```python
from build123d import *

# Parameters (mm, degrees)
SKETCH2_W           = 2.54
SKETCH2_H           = 14.2875
CUT_EXTRUDE1_DEPTH  = 16.757342995
SKETCH3_W           = 1.5875
SKETCH3_H           = 7.9375
SKETCH3_W_2         = 4.7625
SKETCH3_H_2         = 4.7625
BOSS_EXTRUDE2_DEPTH = 3.175
SKETCH4_R           = 1.5875
CUT_EXTRUDE2_DEPTH  = 18.768884025
CHAMFER2_SIZE       = 0.79375
FILLET3_R           = 3.175


with BuildPart() as part:
    # Sketch1 → Revolve1 (revolve)
    with BuildSketch(Plane.XY, mode=Mode.PRIVATE) as revolve1_sk:
        Polygon((1.5875, 7.9375), (1.5875, 0), (3.0988, 0), (3.0988, 6.35), (4.699, 6.35), (4.699, 14.2875), (3.1115, 14.2875), (3.1115, 7.9375), align=None)
    revolve(revolve1_sk.sketch.rotate(Axis((0, 0.120875177, 0), (0, -1, 0)), 180), axis=Axis((0, 0.120875177, 0), (0, -1, 0)))

    # Sketch2 → Cut-Extrude1 (cut, through all)
    with BuildSketch(Plane.XY):
        with Locations((0, 7.14375)):
            Rectangle(SKETCH2_W, SKETCH2_H)
    extrude(amount=CUT_EXTRUDE1_DEPTH, mode=Mode.SUBTRACT)

    # Sketch3 → Boss-Extrude2 (add, symmetric)
    # profile 1 of 3: a face of its own
    with BuildSketch(Plane(origin=(0, 0, 0), x_dir=(0, 0, -1), z_dir=(1, 0, 0))):
        with Locations((3.90525, 10.31875)):
            Rectangle(SKETCH3_W, SKETCH3_H)
    # profile 2 of 3: a face of its own
    with BuildSketch(Plane(origin=(0, 0, 0), x_dir=(0, 0, -1), z_dir=(1, 0, 0))):
        with Locations((7.08025, 10.31875)):
            Rectangle(SKETCH3_W_2, SKETCH3_H)
        with Locations((7.08025, 10.31875)):
            Rectangle(SKETCH3_W, SKETCH3_H_2, mode=Mode.SUBTRACT)
    # profile 3 of 3: a face of its own
    with BuildSketch(Plane(origin=(0, 0, 0), x_dir=(0, 0, -1), z_dir=(1, 0, 0))):
        with Locations((7.08025, 10.31875)):
            Rectangle(SKETCH3_W, SKETCH3_H_2)
    extrude(amount=BOSS_EXTRUDE2_DEPTH, both=True)

    # Sketch4 → Cut-Extrude2 (cut, through all)
    with BuildSketch(Plane(origin=(0, 14.2875, 0), x_dir=(1, 0, 0), z_dir=(0, 1, 0))):
        with Locations(Location((0, 6.2865, 0), (0, 0, 180))):
            Circle(SKETCH4_R)
    extrude(amount=-CUT_EXTRUDE2_DEPTH, mode=Mode.SUBTRACT)

    # Chamfer2
    chamfer2_edges = [part.edges().sort_by_distance(p)[0] for p in [
        (0, 14.2875, -3.1115),
        (0, 0, -3.0988),
        (1.5875, 6.35, -6.2865),
        (1.5875, 14.2875, -6.2865),
    ]]
    chamfer(chamfer2_edges, length=CHAMFER2_SIZE - 0.0001)  # a hair under: the kernel refuses the full size

    # Fillet3
    fillet3_edges = [part.edges().sort_by_distance(p)[0] for p in [
        (3.175, 10.31875, -3.464098151),
        (-3.175, 10.31875, -3.464098151),
        (-3.175, 10.31875, -9.4615),
        (3.175, 10.31875, -9.4615),
    ]]
    fillet(fillet3_edges, radius=FILLET3_R - 0.0001)  # a hair under: the kernel refuses the full size


solid = part.part
```
Check sheet for the modelled part. Datum: model origin and axes. Units: mm. A direction names the side the tool comes from. Coordinates: 2 decimals unless noted, no trailing zeros. Loops run counter-clockwise (first coordinate to the right, second up) from the corner with the lowest first, then second, coordinate; pieces in that order, holes last.
1) Gauge pin test, flat ends, axial feed: pin 1 (4 mm diameter, centred on y = 9.5, z = 2.5, fed in from +X); pin 2 (2 mm diameter, centred on x = -3.5, z = -3.5, fed in from -Y); pin 3 (3 mm diameter, centred on x = 1, y = 9.5, fed in from +Z); pin 4 (3 mm diameter, centred on x = 0, z = 0, fed in from -Y). Record the tip position at first contact, or that the pin passes through.
2) Sectioned sample at C-C (y = 2.25). Record the boundary of the cut face in (x, z) (1 decimal), and give its area (3 significant figures).
3) Release check for a two-part mould opening along Z. For faces 1 (the face through (-3.33, 10.37, -3.68)), 2 (the face through (0.344, 10.363, -7.836)), 3 (the face through (-3.175, 10, -5)) record: released by +Z, released by -Z, zero draft, split by the parting line, or undercut.
4) Sectioned sample at A-A (z = 0). Record the boundary of the cut face in (x, y).
5) Access from +Z, -Z, +X, -X, +Y, -Y to the whole of each face (thin tool, end or side, straight path). Record for faces 4 (the face through (3.33, 10.37, -3.68)), 5 (the face through (-0.118, 3.611, -3.097)), 6 (the face through (-0.12, 10.68, -3.11)), 7 (the face through (-1.27, 7, 3)), 8 (the face through (-4.42, 10.37, 1.59)).
6) Material ranges on probe 1 along Z at (x, y) = (0, 11.25); probe 2 along X at (y, z) = (9.5, 0); probe 3 along X at (y, z) = (3.75, 0), recorded low to high.
Check sheet entries:
1. pin 1: stops at x = 4.67
1. pin 2: stops at y = 6.35
1. pin 3: stops at z = 4.52
1. pin 4: passes through
2. outline: (-1.3, 1) - (-1.3, 2.8) arc R3.1 ccw (long way) to (1.3, 2.8) - (1.3, 1) arc R1.6 cw (long way) to start
2. area: 18.2 mm2
3. face 1: released by -Z
3. face 2: undercut
3. face 3: zero draft
4. outline: (-4.7, 6.35) - (-3.1, 6.35) - (-3.1, 0.79) - (-2.31, 0) - (-1.59, 0) - (-1.59, 7.94) - (-3.11, 7.94) - (-3.11, 13.49) - (-3.91, 14.29) - (-4.7, 14.29) - close; (1.59, 0) - (2.31, 0) - (3.1, 0.79) - (3.1, 6.35) - (4.7, 6.35) - (4.7, 14.29) - (3.91, 14.29) - (3.11, 13.49) - (3.11, 7.94) - (1.59, 7.94) - close
5. face 4: -Z, +X, +Y, -Y
5. face 5: -Y
5. face 6: +Y
5. face 7: +Z, +Y, -Y
5. face 8: -X, +Y, -Y
6. probe 1: z = -9.46 to -7.87, -4.7 to -3.11
6. probe 2: x = -4.7 to -3.11, 3.11 to 4.7
6. probe 3: x = -3.1 to -1.59, 1.59 to 3.1
